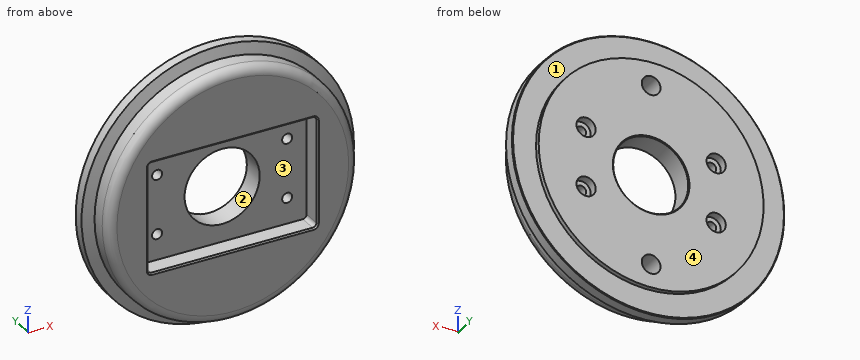
Autodesk Inventor part; units mm, degrees
ref_plane "YZ Plane" through (0, 0, 0) normal (1, 0, 0) x (0, 1, 0)
ref_plane "XZ Plane" through (0, 0, 0) normal (0, 1, 0) x (-1, 0, 0)
ref_plane "XY Plane" through (0, 0, 0) normal (0, 0, 1) x (1, 0, 0)
sketch "Sketch1" plane through (0, 0, 0) normal (0, 0, 1) x (1, 0, 0)
  line L0 (17.5514, 0) -> (46.0756, 0)
  line L1 (46.0756, 0) -> (46.0756, 12.7)
  line L2 (46.0756, 12.7) -> (0, 12.7)
  line L3 (0, 12.7) -> (0, 0)
  line L4 (17.5514, 12.7) -> (17.5514, 0)
  line L5 (46.0756, 8.9662) -> (42.3672, 8.9662)
  line L6 (42.3672, 7.747) -> (42.3672, 0)
  line L7 (46.0756, 7.747) -> (42.3672, 7.747)
  line L8 (46.0756, 8.9662) -> (42.3672, 7.747)
  line L9 (0, 11.1252) -> (0, 12.7)
  line L10 (17.5514, 0) -> (23.85, 0)
  line L11 (0, -2.5) -> (0, 0)
  line L12 (0, 12.7) -> (38.0365, 12.7)
  line L13 (38.0365, 12.7) -> (38.0365, 14.2748)
  line L14 (38.0365, 14.2748) -> (0, 14.2748)
  line L15 (0, 14.2748) -> (0, 12.7)
  line L16 (17.5514, 12.7) -> (17.5514, 14.2748)
  line L17 (0, 0) -> (17.5514, 0)
  dimension "d1" = 12.7
  dimension "d3" = 3.7338
  dimension "d5" = 4.953
  dimension "d8" = 17.5514
  dimension "d9" = 42.3672
  dimension "d10" = 46.0756
  dimension "d11" = 1.5748
  dimension "d12" = 38.0365
revolve "Revolution1" add sketch "Sketch1" angle 360 about axis through (0, 12.7, 0) along (0, -1, 0) contours L4 L2 L1 L8 L6 L0 | L17 L3 L2 L4 | L16 L14 L13 L2 | L2 L15 L14 L16
sketch "Sketch2" plane through (0, 14.2748, 0) normal (0, 1, 0) x (1, 0, 0)
  circle A0 centre (0, 0) radius 30.1752
  point P0 (0, 30.1752)
  point P1 (0, -30.1752)
  dimension "d14" = 60.3504
hole "Hole1" at (0, 14.2748, -30.1752) at (0, 14.2748, 30.1752) direction (0, -1, 0) diameter 6.35 depth 7.62
fillet "Fillet1" radius 3.175 1 edges at (-42.3672, 0, 0)
sketch "Sketch3" plane through (0, 0, 0) normal (0, -1, 0) x (1, 0, 0)
  line L0 (27.305, 18.669) -> (-27.305, 18.669)
  line L1 (-28.575, 17.399) -> (-28.575, -17.399)
  line L2 (-27.305, -18.669) -> (27.305, -18.669)
  line L3 (28.575, -17.399) -> (28.575, 17.399)
  line L4 (28.575, 18.669) -> (-28.575, -18.669) construction
  line L5 (-28.575, 18.669) -> (28.575, -18.669) construction
  arc A0 (27.305, -18.669) -> (28.575, -17.399) centre (27.305, -17.399) ccw
  arc A1 (28.575, 17.399) -> (27.305, 18.669) centre (27.305, 17.399) ccw
  arc A2 (-27.305, 18.669) -> (-28.575, 17.399) centre (-27.305, 17.399) ccw
  arc A3 (-28.575, -17.399) -> (-27.305, -18.669) centre (-27.305, -17.399) ccw
  point P0 (0, 0)
  dimension "d23" = 57.15
  dimension "d24" = 37.338
  dimension "d25" = 1.27
sketch "Sketch4" plane through (0, 14.2748, 0) normal (0, 1, 0) x (1, 0, 0)
  line L0 (21.9964, 9.9949) -> (-21.9964, 9.9949)
  line L1 (-21.9964, 9.9949) -> (-21.9964, -9.9949)
  line L2 (-21.9964, -9.9949) -> (21.9964, -9.9949)
  line L3 (21.9964, -9.9949) -> (21.9964, 9.9949)
  line L4 (21.9964, 9.9949) -> (-21.9964, -9.9949) construction
  line L5 (-21.9964, 9.9949) -> (21.9964, -9.9949) construction
  point P0 (0, 0)
  dimension "d26" = 19.9898
  dimension "d27" = 43.9928
hole "Hole2" at (21.9964, 14.2748, 9.9949) at (21.9964, 14.2748, -9.9949) at (-21.9964, 14.2748, 9.9949) at (-21.9964, 14.2748, -9.9949) direction (0, -1, 0) diameter 3.4036 end through all counterbore diameter 6.5024 counterbore depth 2.9972
extrude "Extrusion1" cut sketch "Sketch3" against normal blind 6.35
chamfer "Chamfer1" distance 0.508 angle 45 8 edges at (0, 0, 18.669) (28.203, 0, 18.297) (28.575, 0, 0) (28.203, 0, -18.297) (0, 0, -18.669) (-28.203, 0, -18.297) (-28.575, 0, 0) (-28.203, 0, 18.297)
sketch "Sketch5" plane through (0, 14.2748, 0) normal (0, 1, 0) x (1, 0, 0)
  circle A0 centre (0, 0) radius 12.7
  dimension "d40" = 25.4
extrude "Extrusion2" cut sketch "Sketch5" against normal through all
chamfer "Chamfer2" distance 0.254 angle 45 2 edges at (-46.0756, 12.7, 0) (-12.7, 14.2748, 0)
properties part number "2016.06.09 ps Hamamatsu PMT Adapter" material "Aluminum 6061"
Source: CAD feature listing. Evaluate the final solid. Frame: model axes, mm. Face numbers are marked on the shaded views. A direction names the side the tool comes from. Round coordinates to 2 decimals unless told otherwise and drop trailing zeros. Loops run counter-clockwise (first coordinate to the right, second up) from the corner with the lowest first, then second, coordinate; pieces in that order, holes last. Notation, with made-up numbers: M 47,-11 L 63,-11 A21 ccw 63,9 Z; hole C -32.5,63 d8. An arc over 180 degrees is marked long. Return JSON: item names as keys, results as strings. Group by question number.
1. Mould query, pull axis X, two halves, no side actions, for the marked faces 1 and 2. Classes: released by +X, released by -X, zero draft, split by the parting line, or undercut.
2. Reachability of the marked faces 3 and 4 from +Z, -Z, +X, -X, +Y, -Y: full face, straight path, thin tool, end or side. Return the list, or none.
3. Section query B-B on y = 4.5. Output: boundary loops of the cut face in (x, z) (3 decimals).
4. Pin query (flat end, axial travel): pin 1 (6 mm diameter, centred on x = 26, y = 4.5, fed in from -Z); pin 2 (5 mm diameter, centred on x = 13, y = 9.5, fed in from +Z); pin 3 (1.8 mm diameter, centred on x = 2, y = 3, fed in from -Z). Return the tip coordinate at first contact, or that it passes through.
5. Material intervals for line 1 along Z through (x, y) = (0, 10.5); line 2 along X through (y, z) = (13.75, -0.5); line 3 along Z through (x, y) = (-22, 11.75), sorted ascending. Write a range as from..to.
Checks:
{
 "1": {"face 1": "zero draft", "face 2": "undercut"},
 "2": {"face 3": "-Y", "face 4": "+Z, -Z, +X, -X, +Y"},
 "3": {"outline": "C 0,0 d84.734; hole M -28.575,-17.399 A1.27 ccw -27.305,-18.669 L 27.305,-18.669 A1.27 ccw 28.575,-17.399 L 28.575,17.399 A1.27 ccw 27.305,18.669 L -27.305,18.669 A1.27 ccw -28.575,17.399 Z"},
 "4": {"pin 1": "stops at z = -35.58", "pin 2": "stops at z = 44.86", "pin 3": "stops at z = -42.35"},
 "5": {"line 1": "z = -46.08..-33.35, -27..-12.7, 12.7..27, 33.35..46.08", "line 2": "x = -38.03..-12.69, 12.69..38.03", "line 3": "z = -40.48..-13.25, -6.74..6.74, 13.25..40.48"}
}
